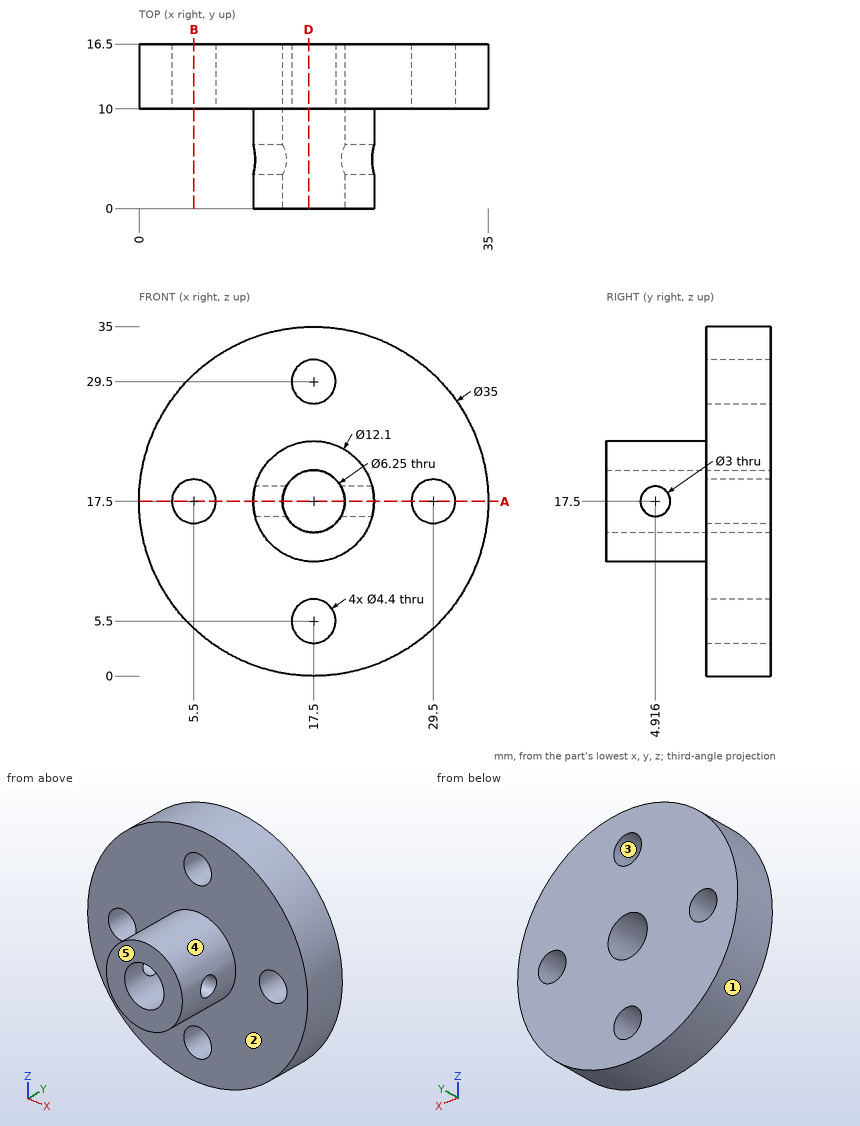
Design review of the part shown in the three views and the two pictorial views. Dimensions are in mm from the part's minimum x, y and z. A direction names the side the tool comes from. Round coordinates to 2 decimals unless told otherwise and drop trailing zeros. Loops run counter-clockwise (first coordinate to the right, second up) from the corner with the lowest first, then second, coordinate; pieces in that order, holes last. Notation, with made-up numbers: (82, 37.25) -> (94, 37.25) arc R17 ccw to (94, 56.25) -> close; hole circle Ø11 at (-40, 55.25). An arc over 180 degrees is marked (long way). Use one line per item in the form item = value. Start each with the question number.
Q1. We need section A-A on z = 17.5. State how many separate pieces and enclosed holes the cut face has, then the cut area to 3 significant figures.
Q2. For pin 1 Ø3.5 at (y, z) = (4.92, 17.5) entering from -X; pin 2 Ø4 at (x, y) = (12, 13) entering from +Z; pin 3 Ø3 at (x, y) = (21, 3.5) entering from -Z, all flat-tipped, find the tip position at first contact; note any pin that passes through.
Q3. Wall thickness on line 1 along X through (y, z) = (14, 17.5) (1 decimal); line 2 along Y through (x, z) = (21.8, 17.5); line 3 along Y through (x, z) = (24.5, 24): over which ranges is each line inside the solid? List them lowest first. Write a range as [from, to].
Q4. Machinability: for the marked faces 4 and 5, which of the approach directions +Z, -Z, +X, -X, +Y, -Y give a long, thin tool a straight path to every point of the face, cutting with its end or side? Answer none if there is none.
Q5. We need section B-B on x = 5.5. Give the boundary of the cut face in (y, z), then the cut area to 3 significant figures.
Q6. Draft analysis for pull direction Z (two halves, no side actions). For the marked faces 1, 2 and 3, state which applies: +Z half, -Z half, draft (parallel to the pull), parting line (faces both ways), or undercut.
Q7. We need section D-D on x = 17. Give the boundary of the cut face in (y, z) (1 decimal).
Calculated:
q1.separate_pieces = 6
q1.enclosed_holes = 0
q1.area = 171 mm²
q2.pin_1 = 11.45
q2.pin_2 = 34.65
q2.pin_3 = 11.79
q3.line_1 = [0, 3.3], [7.7, 14.4], [20.6, 27.3], [31.7, 35]
q3.line_2 = [0, 3.42], [6.42, 16.5]
q3.line_3 = [10, 16.5]
q4.face_4 = -Y
q4.face_5 = +Z, -Z, +X, -X, -Y
q5.outline = (10, 4.76) -> (16.5, 4.76) -> (16.5, 15.3) -> (10, 15.3) -> close; (10, 19.7) -> (16.5, 19.7) -> (16.5, 30.24) -> (10, 30.24) -> close
q5.area = 137 mm²
q6.face_1 = parting line
q6.face_2 = draft
q6.face_3 = undercut
q7.outline = (0, 11.5) -> (10, 11.5) -> (10, 7.6) -> (16.5, 7.6) -> (16.5, 14.4) -> (0, 14.4) -> close; (0, 20.6) -> (16.5, 20.6) -> (16.5, 27.4) -> (10, 27.4) -> (10, 23.5) -> (0, 23.5) -> close; (10, 0) -> (16.5, 0) -> (16.5, 3.4) -> (10, 3.4) -> close; (10, 31.6) -> (16.5, 31.6) -> (16.5, 35) -> (10, 35) -> close
